```python
from build123d import *

# Parameters (mm, degrees)
F0_R      = 1.65
F0_R_2    = 18.5
F1_DEPTH  = 3
F3_DEPTH  = 40
F4_R      = 1.65
F5_DEPTH  = 40.001
F7_DEPTH  = 3
F8_R      = 1.99999
F11_DEPTH = 11
F14_DEPTH = 10.501
F15_SIZE2 = 2
F15_SIZE  = 1
F16_R     = 1


# Not quite as in the source:
# - a fillet or chamfer is up to 0.001 mm smaller than in the source, because OpenCascade refuses the exact size


with BuildPart() as f1:
    # F0 (on Top) → F1 (new body)
    with BuildSketch(Plane.XY):
        with BuildLine():
            Line((40, 0), (0, 0))
            Line((0, 0), (0, -42))
            ThreePointArc((0, -42), (0.8786796564, -44.1213203436), (3, -45))
            Line((3, -45), (37, -45))
            ThreePointArc((37, -45), (39.1213203436, -44.1213203436), (40, -42))
            Line((40, -42), (40, 0))
        make_face()
        with Locations((4, -41)):
            Circle(F0_R, mode=Mode.SUBTRACT)
        with Locations((36, -41)):
            Circle(F0_R, mode=Mode.SUBTRACT)
        with Locations((20, -25)):
            Circle(F0_R_2, mode=Mode.SUBTRACT)
        with Locations((4, -9)):
            Circle(F0_R, mode=Mode.SUBTRACT)
        with Locations((36, -9)):
            Circle(F0_R, mode=Mode.SUBTRACT)
    extrude(amount=F1_DEPTH)

    # F2 (on Right) → F3 (join)
    with BuildSketch(Plane.YZ):
        with BuildLine():
            Line((-2.5, 5), (-2.5, 0))
            Line((-2.5, 0), (7.5, 0))
            Line((7.5, 0), (7.5, 5))
            ThreePointArc((7.5, 5), (2.5, 10), (-2.5, 5))
        make_face()
    extrude(amount=F3_DEPTH)

    # F4 (on face) → F5 (cut, through all)
    with BuildSketch(Plane.YZ.offset(40)):
        with Locations((2.5, 5)):
            Circle(F4_R)
    extrude(amount=-F5_DEPTH, mode=Mode.SUBTRACT)

    # F6 (on face) → F7 (cut)
    with BuildSketch(Plane.YZ.offset(40)):
        Polygon((5.5, 3.2679491924), (5.5, 6.7320508076), (2.5, 8.4641016151), (-0.5, 6.7320508076), (-0.5, 3.2679491924), (2.5, 1.5358983849), align=None)
    extrude(amount=-F7_DEPTH, mode=Mode.SUBTRACT)

    # F8 (radius 2 in the source; OpenCascade refuses exactly that, so slightly less here)
    f8_edges = [f1.edges().sort_by_distance(p)[0] for p in [
        (20, -2.5, 3),
    ]]
    fillet(f8_edges, radius=F8_R)

    # F10 (on offset) → F11 (cut)
    with BuildSketch(Plane.YZ.offset(30.5)):
        with BuildLine():
            Line((8.25, -0.75), (8.25, 5))
            ThreePointArc((8.25, 5), (-1.5658639918, 9.0658639918), (2.5, -0.75))
            Line((2.5, -0.75), (8.25, -0.75))
        make_face()
    extrude(amount=-F11_DEPTH, mode=Mode.SUBTRACT)

    # F13 (on offset) → F14 (cut, through all)
    with BuildSketch(Plane.YZ.offset(10.5)):
        with BuildLine():
            Line((8.25, -0.75), (8.25, 5))
            ThreePointArc((8.25, 5), (-1.5658639918, 9.0658639918), (2.5, -0.75))
            Line((2.5, -0.75), (8.25, -0.75))
        make_face()
    extrude(amount=-F14_DEPTH, mode=Mode.SUBTRACT)

    # F15
    f15_edges = [f1.edges().sort_by_distance(p)[0] for p in [
        (35.25, 7.5, 0),
        (15, 7.5, 0),
    ]]
    f15_side = f1.faces().sort_by_distance((15, 6.839981, 0))[0]
    chamfer(f15_edges, length=F15_SIZE, length2=F15_SIZE2, reference=f15_side)

    # F16
    f16_edges = [f1.edges().sort_by_distance(p)[0] for p in [
        (25, -3.075892, 3.595745),
        (25, -0.339454, 0),
        (5.25, -3.075892, 3.595745),
        (5.25, -0.339454, 0),
    ]]
    fillet(f16_edges, radius=F16_R)


solid = f1.part
```
Part model, mm, in its own coordinate system. A direction names the side the tool comes from. Round coordinates to 2 decimals unless told otherwise and drop trailing zeros. Loops run counter-clockwise (first coordinate to the right, second up) from the corner with the lowest first, then second, coordinate; pieces in that order, holes last.
Item 1: Mould opens along X. For faces 1 (the face through (2.35, -8.93, 1.48)), 2 (the face through (35, 7.5, 3)), 3 (the face through (40, -12.1, 2.8)) say: +X half, -X half, draft (parallel to the pull), parting line (faces both ways), or undercut.
Item 2: Cut at B-B, the plane x = 36. State how many separate pieces and enclosed holes the cut face has, then the cut area to 3 significant figures.
Item 3: Drop flat-ended pins along their axis: P1, Ø3, axis at y = 1.5, z = 2.5, coming from the -X side; P2, Ø1.5, axis at x = 30.5, z = 8.5, coming from the +Y side; P3, Ø2.5, axis at x = 38, z = 4.5, coming from the -Y side; P4, Ø4.5, axis at x = 4, y = -41, coming from the -Z side. Give the stop position or say it passes through.
Item 4: Cut at D-D, the plane z = 4.25. Give the cut face in (x, y), then the cut area to 3 significant figures.
Item 5: 3-axis set-ups, long thin cutter, end or side, ignore diameter. For faces 4 (the face through (34.35, -8.93, 1.48)), 5 (the face through (8, -40, 3)), 6 (the face through (38.5, 1, 7.6)): which of +Z, -Z, +X, -X, +Y, -Y reach the whole face in a straight line?
Item 6: Cut at A-A, the plane y = -25. Give the cut face in (x, z), then the cut area to 3 significant figures.
Item 7: Drill centre lines: line 1 (Y direction, x = 4, z = 1.7); line 2 (X direction, y = 0.5, z = 0.75); line 3 (Y direction, x = 36, z = 0.9). Where is each one in solid material? Low to high.
A:
1. face 1: undercut
1. face 2: draft
1. face 3: +X half
2. separate pieces: 4
2. enclosed holes: 1
2. area: 133 mm2
3. P1: stops at x = 10.5
3. P2: stops at y = 6.68
3. P3: stops at y = -3.53
3. P4: stops at z = 0
4. outline: (10.5, -2.65) - (19.5, -2.65) - (19.5, 1.03) - (10.5, 1.03) - close; (10.5, 3.97) - (19.5, 3.97) - (19.5, 7.5) - (10.5, 7.5) - close; (30.5, -2.65) - (40, -2.65) - (40, -0.5) - (37, -0.5) - (37, 1.03) - (30.5, 1.03) - close; (30.5, 3.97) - (37, 3.97) - (37, 5.5) - (40, 5.5) - (40, 7.5) - (30.5, 7.5) - close
4. area: 124 mm2
5. face 4: +Z, -Z
5. face 5: +Z, +X, -X, -Y
5. face 6: +X
6. outline: (0, 0) - (1.5, 0) - (1.5, 3) - (0, 3) - close; (38.5, 0) - (40, 0) - (40, 3) - (38.5, 3) - close
6. area: 9.00 mm2
7. line 1: y = -45 to -42.65, -39.35 to -34.29, -15.71 to -10.65, -7.35 to -2.21
7. line 2: x = 10.5 to 19.5, 30.5 to 40
7. line 3: y = -45 to -42.65, -39.35 to -34.29, -15.71 to -10.65, -7.35 to 6.95
